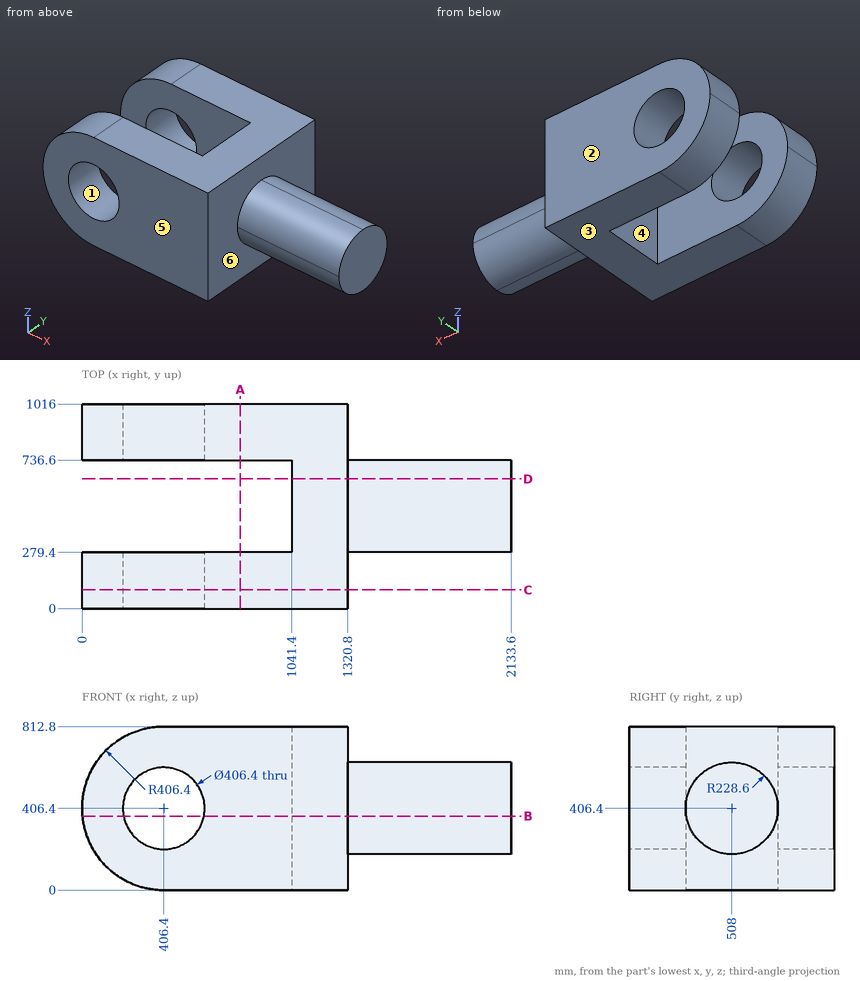
Can you work these out from the drawing? Everything is in mm from the part's minimum corner. A direction names the side the tool comes from. Coordinates: 2 decimals unless noted, no trailing zeros. Order: outer loops, then holes, each group sorted by start corner. A loop starts at its lowest first (then second) coordinate and runs counter-clockwise, first axis right, second up. Notation, with made-up numbers: M -21,72.25 L -5,72.25 A37 ccw -5,108.25 Z; hole C 23,-28.75 d10. An arc over 180 degrees is marked long. Answer as CSV lines item,"result". Start each with the question number.
1. I want a section at A-A, the plane x = 787. Write out the boundary of the cut face in (y, z), and give its area (3 significant figures).
2. We'd pull the mould along Z, two halves only. Please class the marked faces 1, 2 and 3: released by +Z, released by -Z, zero draft, split by the parting line, or undercut.
3. I want a section at D-D, the plane y = 644. Write out the boundary of the cut face in (x, z).
4. I want a section at B-B, the plane z = 367. Write out the boundary of the cut face in (x, y).
5. I want a section at C-C, the plane y = 92. Write out the boundary of the cut face in (x, z), and give its area (3 significant figures).
6. For pin 1 (1.5 mm diameter, centred on y = 782.5, z = 347.5, fed in from -X); pin 2 (8 mm diameter, centred on y = 139, z = 397.5, fed in from +X); pin 3 (12 mm diameter, centred on x = 1905, y = 597, fed in from +Z), each with a flat end and sliding along its axis, tell me the tip position at first contact or that it passes through.
7. I need wall thicknesses on line 1 (Z direction, x = 406.4, y = 813.5); line 2 (Y direction, x = 800, z = 430.5); line 3 (X direction, y = 420.5, z = 571). Which ranges of each line are inside material? Lowest first, please. Write a range as [from, to].
8. On a 3-axis mill with a long thin cutter (end or side, diameter ignored), from which of +Z, -Z, +X, -X, +Y, -Y can I reach the whole of each face in a straight line? I mean the marked faces 4, 5 and 6. Say none if no direction works.
Recorded:
1,outline,"M 0,0 L 279.4,0 L 279.4,812.8 L 0,812.8 Z; M 736.6,0 L 1016,0 L 1016,812.8 L 736.6,812.8 Z"
1,area,"454,000 mm2"
2,face 1,"undercut"
2,face 2,"zero draft"
2,face 3,"released by -Z"
3,outline,"M 1041.4,0 L 1320.8,0 L 1320.8,222.66 L 2133.6,222.66 L 2133.6,590.14 L 1320.8,590.14 L 1320.8,812.8 L 1041.4,812.8 Z"
4,outline,"M 1.91,0 L 207.06,0 L 207.06,279.4 L 1.91,279.4 Z; M 1.91,736.6 L 207.06,736.6 L 207.06,1016 L 1.91,1016 Z; M 605.74,0 L 1320.8,0 L 1320.8,282.82 L 2133.6,282.82 L 2133.6,733.18 L 1320.8,733.18 L 1320.8,1016 L 605.74,1016 L 605.74,736.6 L 1041.4,736.6 L 1041.4,279.4 L 605.74,279.4 Z"
5,outline,"M 406.4,0 L 1320.8,0 L 1320.8,812.8 L 406.4,812.8 A406.4 ccw Z; hole C 406.4,406.4 d406.4"
5,area,"873,000 mm2"
6,pin 1,"stops at x = 4.18"
6,pin 2,"stops at x = 1320.8"
6,pin 3,"stops at z = 619.4"
7,line 1,"z = [0, 203.2], [609.6, 812.8]"
7,line 2,"y = [0, 279.4], [736.6, 1016]"
7,line 3,"x = [1041.4, 2133.6]"
8,face 4,"+Z, -Z, -X"
8,face 5,"+Z, -Z, +X, -X, -Y"
8,face 6,"+X"
